from build123d import *

# Parameters (mm, degrees)
F0_R     = 19
F1_DEPTH = 40
F2_R     = 19
F3_DEPTH = 25


with BuildPart() as f1:
    # F0 (on Front) → F1 (new body)
    with BuildSketch(Plane.XZ):
        with BuildLine():
            ThreePointArc((0, 0), (15.202796, 6.297204), (21.5, 21.5))
            ThreePointArc((21.5, 21.5), (0, 43), (-21.5, 21.5))
            ThreePointArc((-21.5, 21.5), (-15.202796, 6.297204), (0, 0))
        make_face()
        with Locations((0, 21.5)):
            Circle(F0_R, mode=Mode.SUBTRACT)
        with BuildLine():
            Line((21.5, 0), (21.5, 21.5))
            ThreePointArc((21.5, 21.5), (15.202796, 6.297204), (0, 0))
            Line((0, 0), (21.5, 0))
        make_face()
        with BuildLine():
            ThreePointArc((0, 0), (-15.202796, 6.297204), (-21.5, 21.5))
            Line((-21.5, 21.5), (-21.5, 0))
            Line((-21.5, 0), (0, 0))
        make_face()
    extrude(amount=F1_DEPTH)

    # F2 (on face) → F3 (join)
    with BuildSketch(Plane(origin=(0, 0, 0), x_dir=(1, 0, 0), z_dir=(0, 0, -1))):
        with Locations((0, 20)):
            Circle(F2_R)
    extrude(amount=F3_DEPTH)


solid = f1.part
Here's how the part is built. I have some questions about the finished solid (model axes, mm). A direction names the side the tool comes from. Round coordinates to 2 decimals unless told otherwise and drop trailing zeros. Order: outer loops, then holes, each group sorted by start corner. A loop starts at its lowest first (then second) coordinate and runs counter-clockwise, first axis right, second up. Notation, with made-up numbers: (32, 13) -> (36, 13) arc R26 ccw to (36, 40) -> close; hole circle Ø9 at (66, -21). An arc over 180 degrees is marked (long way). Use CSV: the item, a comma, the result in double quotes.
1. I want a section at C-C on z = 6. List the corners of the cut face in (x, y) for me.
Recorded:
outline,"(-21.5, -40) -> (-10.99, -40) -> (-10.99, 0) -> (-21.5, 0) -> close; (10.99, -40) -> (21.5, -40) -> (21.5, 0) -> (10.99, 0) -> close"
2. I want a section at B-B on x = 0. List the corners of the cut face in (y, z) for me.
Recorded:
outline,"(-40, 0) -> (-39, 0) -> (-39, -25) -> (-1, -25) -> (-1, 0) -> (0, 0) -> (0, 2.5) -> (-40, 2.5) -> close; (-40, 40.5) -> (0, 40.5) -> (0, 43) -> (-40, 43) -> close"
3. I want a section at D-D on x = 5.5. List the corners of the cut face in (y, z) for me, and give its area (3 significant figures).
Recorded:
outline,"(-40, 0) -> (-38.19, 0) -> (-38.19, -25) -> (-1.81, -25) -> (-1.81, 0) -> (0, 0) -> (0, 3.31) -> (-40, 3.31) -> close; (-40, 39.69) -> (0, 39.69) -> (0, 42.28) -> (-40, 42.28) -> close"
area,"1,150 mm2"
4. Which directions (+Z, -Z, +X, -X, +Y, -Y) give clear straight access to the entire face, cutting with the end or side of a thin tool? Please do faces 4 (the face through (-18, -27, 0)), 5 (the face through (-21.5, -20, 11)).
Recorded:
face 4,"-Z"
face 5,"+Z, -Z, -X, +Y, -Y"
5. I'm going to push flat-ended pins straight in: P1, Ø1, axis at y = -12, z = -5, coming from the -X side; P2, Ø1.5, axis at y = -24.5, z = -2, coming from the -X side; P3, Ø10, axis at x = -8, y = -26.5, coming from the +Z side. Where does each tip first touch, or does it pass through?
Recorded:
P1,"stops at x = -17.46"
P2,"stops at x = -18.63"
P3,"stops at z = 42.79"
6. I want a section at A-A on y = -20. List the corners of the cut face in (x, z) for me, and give its area (3 significant figures).
Recorded:
outline,"(-21.5, 0) -> (-19, 0) -> (-19, -25) -> (19, -25) -> (19, 0) -> (21.5, 0) -> (21.5, 21.5) arc R21.5 ccw to (-21.5, 21.5) -> close; hole circle Ø38 at (0, 21.5)"
area,"1,470 mm2"
7. I need wall thicknesses on line 1 along X through (y, z) = (-15, 21); line 2 along Z through (x, y) = (-6.5, -18.5); line 3 along X through (y, z) = (-3.5, 31). Which ranges of each line are inside material? Lowest first, please.
Recorded:
line 1,"x = -21.5 to -18.99, 18.99 to 21.5"
line 2,"z = -25 to 3.65, 39.35 to 41.99"
line 3,"x = -19.29 to -16.45, 16.45 to 19.29"
8. Thinking about a two-plate mould opening in Z: for faces 1 (the face through (10.214, -19.72, 37.521)), 2 (the face through (10.214, -36.021, -12.325)), 3 (the face through (0, -20, -25)), which applies, pulls with the +Z half, pulls with the -Z half, needs draft (parallel to the pull), parting line crosses it, or undercut?
Recorded:
face 1,"undercut"
face 2,"needs draft"
face 3,"pulls with the -Z half"
